The listing builds one solid part. Answer for the finished solid, in the listing's coordinates (mm). A direction names the side the tool comes from. Coordinates: 2 decimals unless noted, no trailing zeros. Order: outer loops, then holes, each group sorted by start corner. A loop starts at its lowest first (then second) coordinate and runs counter-clockwise, first axis right, second up. Notation, with made-up numbers: (36, 19.25) - (67, 19.25) arc R23 cw to (67, 46.25) - close; hole circle Ø2 at (-15.5, 20). An arc over 180 degrees is marked (long way). Use a Markdown table: item, result. Add a question column.
Item 1: The mould has two halves that part along Y. Classify faces 1 (the flat face through (9.3, 20, 2.7)), 2 (the cylindrical face through (10.098, 12.915, 3.935)), 3 (the flat face through (-8.53, 3.94, -6.9)): released by +Y, released by -Y, zero draft, split by the parting line, or undercut.
Item 2: The part is cut by section B-B, the plane y = 7. Give the vertices of the cut face in (x, z), then the cut area to 3 significant figures.
Item 3: Flat-ended cylindrical pins translate along their axes: P1, Ø1, axis at x = 6, y = 12.5, coming from the +Z side (3 decimals); P2, Ø10, axis at x = -3, z = -1, coming from the +Y side; P3, Ø2, axis at x = 7, z = -7, coming from the -Y side; P4, Ø3, axis at x = -3, y = 6, coming from the -Z side. Find the tip coordinate at first contact, or state that the pin passes through.
Item 4: The part is cut by section C-C, the plane x = 0. Give the vertices of the cut face in (y, z), then the cut area to 3 significant figures.
Item 5: The part is cut by section A-A, the plane z = 0. Give the vertices of the cut face in (x, y).
Item 6: For faces 4 (the flat face through (-8.571, 3.944, 6.917)), 5 (the flat face through (-10.808, 3.944, 1.892)), 6 (the flat face through (8.53, 3.94, -6.9)), determine the directions among +Z, -Z, +X, -X, +Y, -Y from which every point of the face is accessible in a straight line to the end or side of a thin tool.
Item 7: Find the intervals of material crossed by line 1 along X through (y, z) = (10, 0); line 2 along Y through (x, z) = (-10, 4.5); line 3 along X through (y, z) = (8.5, 7.25), in increasing order.
Item 8: The part is cut by section D-D, the plane y = 9.75. Give the vertices of the cut face in (x, z).
from build123d import *

# Parameters (mm, degrees)
SKETCH1_R               = 12.5
SKETCH1_R_2             = 9.5
BOSS_EXTRUDE1_DEPTH     = 20
CUT_EXTRUDE1_DEPTH      = 25.498499593
CUT_EXTRUDE1_DEPTH_BACK = 25.498499593
SKETCH2_R               = 2.75
CUT_EXTRUDE2_DEPTH      = 41.591596454
CUT_EXTRUDE2_DEPTH_BACK = 41.591596454
SKETCH3_R               = 2.75
CUT_EXTRUDE3_DEPTH      = 8


with BuildPart() as part:
    # Sketch1 → Boss-Extrude1 (new body)
    with BuildSketch(Plane(origin=(0, 0, 0), x_dir=(1, 0, 0), z_dir=(0, 1, 0))):
        with Locations(Location((0, 0, 0), (0, 0, 270))):
            Circle(SKETCH1_R)
        with Locations(Location((0, 0, 0), (0, 0, 270))):
            Circle(SKETCH1_R_2, mode=Mode.SUBTRACT)
    extrude(amount=BOSS_EXTRUDE1_DEPTH)

    # Sketch2 → Cut-Extrude1 (cut, two sides: drawn at the far end of the back side and taken through both)
    with BuildSketch(Plane(origin=(0, 3.038971661, 0), x_dir=(0.41379310344827586, 0, 0.9103709505133852), z_dir=(-0.9103709505133852, 0, 0.41379310344827586)).offset(-CUT_EXTRUDE1_DEPTH_BACK)):
        with Locations((0, 12.561028339)):
            Circle(SKETCH2_R)
    extrude(amount=CUT_EXTRUDE1_DEPTH + CUT_EXTRUDE1_DEPTH_BACK, mode=Mode.SUBTRACT)

    # Sketch3 → Cut-Extrude2 (cut, two sides: drawn at the far end of the back side and taken through both)
    with BuildSketch(Plane(origin=(-18.02534482, 3.038971661, -8.193103448), x_dir=(-0.41379310344827586, 0, 0.9103709505133852), z_dir=(-0.9103709505133852, 0, -0.41379310344827586)).offset(-CUT_EXTRUDE2_DEPTH_BACK)):
        with Locations((0, 12.561028339)):
            Circle(SKETCH3_R)
    extrude(amount=CUT_EXTRUDE2_DEPTH + CUT_EXTRUDE2_DEPTH_BACK, mode=Mode.SUBTRACT)

    # Sketch6 → Cut-Extrude3 (cut)
    with BuildSketch(Plane(origin=(0, 0, 0), x_dir=(1, 0, 0), z_dir=(0, 1, 0))):
        with BuildLine():
            Line((-9.962903285, -7.549209106), (-7.140314851, -6.266251179))
            ThreePointArc((-7.140314851, -6.266251179), (-8.64852403, -3.931034483), (-9.41617692, -1.259210951))
            Line((-9.41617692, -1.259210951), (-12.238765354, -2.542168878))
            ThreePointArc((-12.238765354, -2.542168878), (-11.379636881, -5.172413793), (-9.962903285, -7.549209106))
        make_face()
        with BuildLine():
            Line((-12.238765354, 2.542168878), (-9.41617692, 1.259210951))
            ThreePointArc((-9.41617692, 1.259210951), (-8.64852403, 3.931034483), (-7.140314851, 6.266251179))
            Line((-7.140314851, 6.266251179), (-9.962903285, 7.549209106))
            ThreePointArc((-9.962903285, 7.549209106), (-11.379636881, 5.172413793), (-12.238765354, 2.542168878))
        make_face()
        with BuildLine():
            Line((7.140314851, 6.266251179), (9.962903285, 7.549209106))
            ThreePointArc((9.962903285, 7.549209106), (11.379636881, 5.172413793), (12.238765354, 2.542168878))
            Line((12.238765354, 2.542168878), (9.41617692, 1.259210951))
            ThreePointArc((9.41617692, 1.259210951), (8.64852403, 3.931034483), (7.140314851, 6.266251179))
        make_face()
        with BuildLine():
            Line((7.140314851, -6.266251179), (9.962903285, -7.549209106))
            ThreePointArc((9.962903285, -7.549209106), (11.379636881, -5.172413793), (12.238765354, -2.542168878))
            Line((12.238765354, -2.542168878), (9.41617692, -1.259210951))
            ThreePointArc((9.41617692, -1.259210951), (8.64852403, -3.931034483), (7.140314851, -6.266251179))
        make_face()
    extrude(amount=CUT_EXTRUDE3_DEPTH, mode=Mode.SUBTRACT)


solid = part.part
Solution:
| question | item | result |
|---|---|---|
| 1 | face 1 | released by +Y |
| 1 | face 2 | undercut |
| 1 | face 3 | zero draft |
| 2 | outline | (-12.24, -2.54) - (-9.42, -1.26) arc R9.5 cw to (-9.42, 1.26) - (-12.24, 2.54) arc R12.5 ccw to start; (-9.96, -7.55) arc R12.5 ccw to (9.96, -7.55) - (7.14, -6.27) arc R9.5 cw to (-7.14, -6.27) - close; (-9.96, 7.55) - (-7.14, 6.27) arc R9.5 cw to (7.14, 6.27) - (9.96, 7.55) arc R12.5 ccw to start; (9.42, -1.26) - (12.24, -2.54) arc R12.5 ccw to (12.24, 2.54) - (9.42, 1.26) arc R9.5 cw to start |
| 2 | area | 141 mm2 |
| 3 | P1 | stops at z = 11.225 |
| 3 | P2 | passes through |
| 3 | P3 | stops at y = 0 |
| 3 | P4 | stops at z = -12.41 |
| 4 | outline | (0, -12.5) - (20, -12.5) - (20, -9.5) - (0, -9.5) - close; (0, 9.5) - (20, 9.5) - (20, 12.5) - (0, 12.5) - close |
| 4 | area | 120 mm2 |
| 5 | outline | (-12.5, 0) - (-9.5, 0) - (-9.5, 20) - (-12.5, 20) - close; (9.5, 0) - (12.5, 0) - (12.5, 20) - (9.5, 20) - close |
| 6 | face 4 | -X, -Y |
| 6 | face 5 | -Y |
| 6 | face 6 | +X, -Y |
| 7 | line 1 | x = -12.5 to -9.5, 9.5 to 12.5 |
| 7 | line 2 | y = 8 to 12.85, 18.35 to 20 |
| 7 | line 3 | x = -10.18 to -6.14, 6.14 to 10.18 |
| 8 | outline | circle Ø25 at (0, 0); hole circle Ø19 at (0, 0) |
